Build history of the part. All positions in model axes, mm. Face numbers are marked on the shaded views. A direction names the side the tool comes from. Give positions to 0.01 mm unless a question says otherwise; leave off trailing zeros. Order: outer loops, then holes, each group sorted by start corner. A loop starts at its lowest first (then second) coordinate and runs counter-clockwise, first axis right, second up. Notation, with made-up numbers: M 53.25,-20.5 L 90.25,-20.5 A11 cw 90.25,0.5 Z; hole C 72,78 d5. An arc over 180 degrees is marked long. One line per item, written item: value.
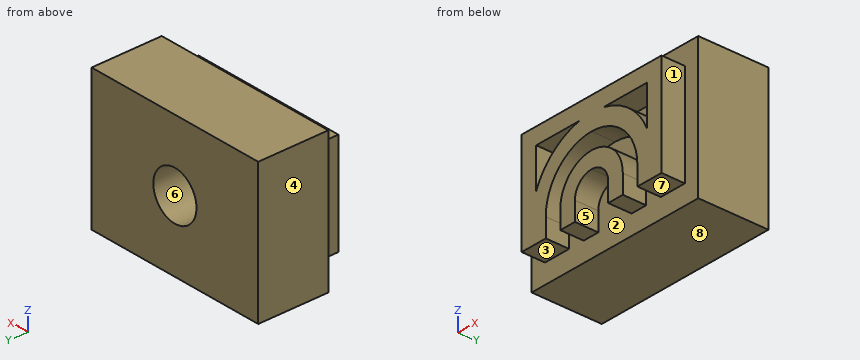
from build123d import *

# Parameters (mm, degrees)
F0_W     = 25.4
F0_H     = 19.05
F1_DEPTH = 9.525
F3_DEPTH = 3.175
F5_D     = 6.5786
F5_DEPTH = 6.35
F5_TIP   = 1.9764108342


with BuildPart() as f1:
    # F0 (on Front) → F1 (new body)
    with BuildSketch(Plane.XZ):
        Rectangle(F0_W, F0_H)
    extrude(amount=-F1_DEPTH)

    # F2 (on face) → F3 (join)
    with BuildSketch(Plane.XZ):
        with BuildLine():
            Line((10.6646052337, 6.8961), (0, 6.8961))
            Line((0, 6.8961), (-10.6646052337, 6.8961))
            Line((-10.6646052337, 6.8961), (-10.6646052337, -6.8961))
            Line((-10.6646052337, -6.8961), (-6.985, -6.8961))
            Line((-6.985, -6.8961), (-6.985, -4.3561))
            ThreePointArc((-6.985, -4.3561), (-4.9391408666, 0.5830408666), (0, 2.6289))
            ThreePointArc((0, 2.6289), (4.9391408666, 0.5830408666), (6.985, -4.3561))
            Line((6.985, -4.3561), (6.985, -6.8961))
            Line((6.985, -6.8961), (10.6646052337, -6.8961))
            Line((10.6646052337, -6.8961), (10.6646052337, 6.8961))
        make_face()
        with BuildLine():
            ThreePointArc((-1.8007149025, 4.6736), (-5.7789138794, 2.8120385746), (-8.4421052337, -0.6806523438))
            Line((-8.4421052337, -0.6806523438), (-8.4421052337, 4.6736))
            Line((-8.4421052337, 4.6736), (-1.8007149025, 4.6736))
        make_face(mode=Mode.SUBTRACT)
        with BuildLine():
            ThreePointArc((8.4421052337, -0.6806523438), (5.7789138794, 2.8120385746), (1.8007149025, 4.6736))
            Line((1.8007149025, 4.6736), (8.4421052337, 4.6736))
            Line((8.4421052337, 4.6736), (8.4421052337, -0.6806523438))
        make_face(mode=Mode.SUBTRACT)
        with BuildLine():
            Line((2.54, -4.3561), (2.54, -6.8961))
            Line((2.54, -6.8961), (4.7625, -6.8961))
            Line((4.7625, -6.8961), (4.7625, -4.3561))
            ThreePointArc((4.7625, -4.3561), (3.3675960454, -0.9885039546), (0, 0.4064))
            ThreePointArc((0, 0.4064), (-3.3675960454, -0.9885039546), (-4.7625, -4.3561))
            Line((-4.7625, -4.3561), (-4.7625, -6.8961))
            Line((-4.7625, -6.8961), (-2.54, -6.8961))
            Line((-2.54, -6.8961), (-2.54, -4.3561))
            ThreePointArc((-2.54, -4.3561), (-1.7960512242, -2.5600487758), (0, -1.8161))
            ThreePointArc((0, -1.8161), (1.7960512242, -2.5600487758), (2.54, -4.3561))
        make_face()
    extrude(amount=F3_DEPTH)

    # F5
    with Locations(Plane(origin=(0, 9.525, 0), x_dir=(-1, 0, 0), z_dir=(0, 1, 0))):
        with Locations((0, 0)):
            Hole(F5_D / 2, depth=F5_DEPTH)
            with Locations((0, 0, -(F5_DEPTH + F5_TIP / 2))):  # 118° drill point
                Cone(0, F5_D / 2, F5_TIP, mode=Mode.SUBTRACT)


solid = f1.part
1) Tool access for the marked faces 5, 6, 7 and 8: list every direction of +Z, -Z, +X, -X, +Y, -Y with a clear straight run to the whole face (end or side of a thin tool).
Check values:
face 5: -Z, -Y
face 6: +Y
face 7: -Z, +X, -X, -Y
face 8: -Z, +X, -X, +Y, -Y
2) Mould opens along X. For the marked faces 1, 2, 3 and 4 say: released by +X, released by -X, zero draft, split by the parting line, or undercut.
Check values:
face 1: released by +X
face 2: undercut
face 3: zero draft
face 4: released by -X
3) Drill centre lines: probe 1 along Z at (x, y) = (0, 6.25) (3 decimals); probe 2 along Z at (x, y) = (-2.75, 4.25) (3 decimals); probe 3 along X at (y, z) = (5.5, 0). Where is each one in solid material? Low to high. Write a range as from..to.
Check values:
probe 1: -9.525..-3.289, 3.289..9.525
probe 2: -9.525..-1.805, 1.805..9.525
probe 3: -12.7..-3.29, 3.29..12.7
4) Saw through at B-B, the plane x = 9.5. Write the cut outline in (y, z) (3 decimals).
Check values:
outline: M -3.175,-6.896 L 0,-6.896 L 0,-9.525 L 9.525,-9.525 L 9.525,9.525 L 0,9.525 L 0,6.896 L -3.175,6.896 Z
5) Saw through at A-A, the plane z = -5.25. Write the cut outline in (x, y) (1 decimal).
Check values:
outline: M -12.7,0 L -10.7,0 L -10.7,-3.2 L -7,-3.2 L -7,0 L -4.8,0 L -4.8,-3.2 L -2.5,-3.2 L -2.5,0 L 2.5,0 L 2.5,-3.2 L 4.8,-3.2 L 4.8,0 L 7,0 L 7,-3.2 L 10.7,-3.2 L 10.7,0 L 12.7,0 L 12.7,9.5 L -12.7,9.5 Z
6) Pin check, flat tips, straight feed: pin 1 (2.5 mm diameter, centred on x = 9.5, y = -1.5, fed in from -Z); pin 2 (4 mm diameter, centred on x = 0, z = 0, fed in from +Y); pin 3 (1 mm diameter, centred on y = -1.5, z = 3.5, fed in from -X). Stop position of each tip, or through.
Check values:
pin 1: z = -6.9
pin 2: y = 2.4
pin 3: x = -10.66
7) Saw through at C-C, the plane y = 4.75. Write the cut outline in (x, z) (3 decimals), then the cut area to 3 significant figures.
Check values:
outline: M -12.7,-9.525 L 12.7,-9.525 L 12.7,9.525 L -12.7,9.525 Z; hole C 0,0 d6.579
area: 450 mm^2
